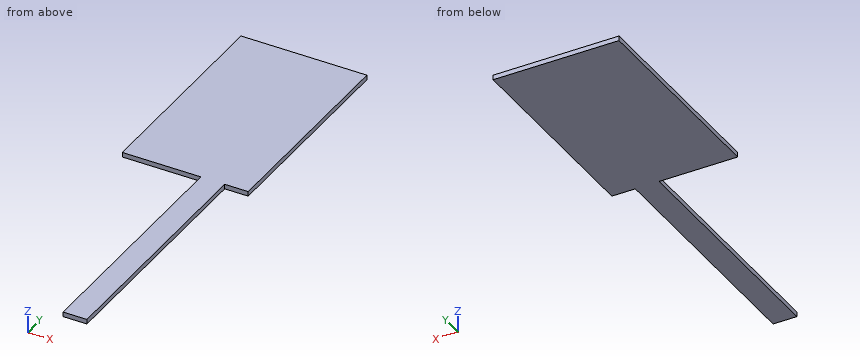
Autodesk Inventor part; units mm, degrees
ref_plane "YZ Plane" through (0, 0, 0) normal (1, 0, 0) x (0, 1, 0)
ref_plane "XZ Plane" through (0, 0, 0) normal (0, 1, 0) x (-1, 0, 0)
ref_plane "XY Plane" through (0, 0, 0) normal (0, 0, 1) x (1, 0, 0)
sketch "Esboço1" plane through (0, 0, 0) normal (0, 0, 1) x (1, 0, 0)
  line L0 (-37.1093, 20.0517) -> (-10.6595, 20.0517)
  line L1 (-10.6595, 20.0517) -> (-37.1093, 20.0517)
  line L2 (-10.6595, 20.0517) -> (-10.6595, -24.2254)
  line L3 (-10.6595, -24.2254) -> (-15.5932, -24.2254)
  line L4 (-15.5932, -24.2254) -> (-15.5932, -75.6194)
  line L5 (-15.5932, -24.2254) -> (-15.5932, -75.6194)
  line L6 (-15.5932, -75.6194) -> (-20.5932, -75.6194)
  line L7 (-20.5932, -75.6194) -> (-20.5932, -24.2254)
  line L8 (-20.5932, -75.6194) -> (-20.5932, -24.2254)
  line L9 (-20.5932, -24.2254) -> (-37.1093, -24.2254)
  line L10 (-20.5932, -24.2254) -> (-37.1093, -24.2254)
  line L11 (-37.1093, -24.2254) -> (-37.1093, 20.0517)
  point P0 (0, 0)
  point P1 (0, 0)
extrude "Extrusão1" add sketch "Esboço1" along normal blind 1
properties part number "Tampa de trás 10-06-2016"
Input: part model. Units: mm. Frame: model coordinates. Coordinates: 2 decimals unless noted, no trailing zeros. Order: outer loops, then holes, each group sorted by start corner. A loop starts at its lowest first (then second) coordinate and runs counter-clockwise, first axis right, second up. Notation, with made-up numbers: M 1,27 L 55,27 A33 cw 55,58 Z; hole C -15,-10 d7. An arc over 180 degrees is marked long. One line per question, with ' | ' between items.
Item 1: Pin query (flat end, axial travel): pin 1 (0.5 mm diameter, centred on x = -30.5, z = 0.5, fed in from -Y). Return the tip coordinate at first contact, or that it passes through.
Geometry results:
pin 1: stops at y = -24.23
Item 2: Section B-B (y = -35). Output: boundary loops of the cut face in (x, z), then the cut area to 3 significant figures.
Geometry results:
outline: M -20.59,0 L -15.59,0 L -15.59,1 L -20.59,1 Z | area: 5.00 mm^2
Item 3: Section A-A (z = 0.25). Output: boundary loops of the cut face in (x, y), then the cut area to 3 significant figures.
Geometry results:
outline: M -37.11,-24.23 L -20.59,-24.23 L -20.59,-75.62 L -15.59,-75.62 L -15.59,-24.23 L -10.66,-24.23 L -10.66,20.05 L -37.11,20.05 Z | area: 1,430 mm^2
Item 4: Section C-C (x = -12.75). Output: boundary loops of the cut face in (y, z), then the cut area to 3 significant figures.
Geometry results:
outline: M -24.23,0 L 20.05,0 L 20.05,1 L -24.23,1 Z | area: 44.3 mm^2
Item 5: Ray query, line 1 along Y through (x, z) = (-34.75, 0.65); line 2 along X through (y, z) = (-38, 0.85). Return the intervals inside material, ascending.
Geometry results:
line 1: y = -24.23 to 20.05 | line 2: x = -20.59 to -15.59
